```python
from build123d import *

# Parameters (mm, degrees)
SKETCH1_R           = 1.9
SKETCH1_R_2         = 1.2
BOSS_EXTRUDE1_DEPTH = 3.5
SKETCH2_R           = 5.9
SKETCH2_R_2         = 4.9
BOSS_EXTRUDE2_DEPTH = 1.5
BOSS_EXTRUDE3_DEPTH = 0.125
CIRPATTERN1_COUNT   = 3


with BuildPart() as part:
    # Sketch1 → Boss-Extrude1 (new body)
    with BuildSketch(Plane.XY):
        Circle(SKETCH1_R)
        Circle(SKETCH1_R_2, mode=Mode.SUBTRACT)
    extrude(amount=BOSS_EXTRUDE1_DEPTH)



with BuildPart() as body_2:
    # Sketch2 → Boss-Extrude2 (new body)
    with BuildSketch(Plane.XY.offset(3.5)):
        Circle(SKETCH2_R)
        Circle(SKETCH2_R_2, mode=Mode.SUBTRACT)
    extrude(amount=-BOSS_EXTRUDE2_DEPTH)


with BuildPart() as part_1:
    add(part.part)

    add(body_2.part)  # Boss-Extrude3 merges body 2
    # Sketch7 → Boss-Extrude3 (add, symmetric)
    with BuildSketch(Plane(origin=(0, 0, 0), x_dir=(0, 0, -1), z_dir=(1, 0, 0))):
        Polygon((-3.498505426, 1.898798754), (-3.498505426, 4.906659039), (-2.003497041, 4.906659039), (0, 1.898798754), (0, 1.698798754), (-3.498505426, 1.698798754), align=None)
    boss_extrude3 = extrude(amount=BOSS_EXTRUDE3_DEPTH, both=True)

    # CirPattern1: Boss-Extrude3 ×3 about axis
    cirpattern1_axis = Axis((0, 0, 0), (0, 0, 1))
    for i in range(1, CIRPATTERN1_COUNT):
        add(boss_extrude3.rotate(cirpattern1_axis, i * 360 / CIRPATTERN1_COUNT))


solid = part_1.part
```
Work out the finished part from the listing and answer in its coordinate system (mm). A direction names the side the tool comes from. Coordinates: 2 decimals unless noted, no trailing zeros. Order: outer loops, then holes, each group sorted by start corner. A loop starts at its lowest first (then second) coordinate and runs counter-clockwise, first axis right, second up. Notation, with made-up numbers: M 89,77.25 L 119,77.25 A13 ccw 119,89.25 Z; hole C 79.25,61.25 d1. An arc over 180 degrees is marked long. Use CSV: the item, a comma, the result in double quotes.
1) Section C-C on z = 0.65 is taken. Write down the section's boundary in (x, y) (3 decimals).
Worked out:
outline,"M -2.552,-1.329 L -2.427,-1.546 L -1.579,-1.056 A1.9 ccw 1.579,-1.056 L 2.427,-1.546 L 2.552,-1.329 L 1.704,-0.84 A1.9 ccw 0.125,1.896 L 0.125,2.875 L -0.125,2.875 L -0.125,1.896 A1.9 ccw -1.704,-0.84 Z; hole C 0,0 d2.4"
2) Section A-A on y = 2.25 is taken. Count the separate pieces of the cut face and the enclosed holes in it, plus the area to 3 significant figures.
Worked out:
separate pieces,"3"
enclosed holes,"0"
area,"4.12 mm^2"
3) Consider line 1 (Y direction, x = 0, z = 2.7); line 2 (Y direction, x = -1, z = 2.95); line 3 (X direction, y = -1.5, z = 1.5). Determine where each line is inside the solid, lowest interval first. Write a range as [from, to].
Worked out:
line 1,"y = [-5.9, -4.9], [-1.9, -1.2], [1.2, 5.9]"
line 2,"y = [-5.81, -4.8], [-1.62, -0.66], [0.66, 1.62], [4.8, 5.81]"
line 3,"x = [-2.85, -2.35], [-1.17, 1.17], [2.35, 2.85]"
4) Determine the mould class of faces 1 (the face through (-5.894, 0.259, 2.76)), 2 (the face through (-1.9, 0.08, 1.73)), 3 (the face through (1, 5, 2)) for opening direction X: released by +X, released by -X, zero draft, split by the parting line, or undercut.
Worked out:
face 1,"split by the parting line"
face 2,"undercut"
face 3,"zero draft"
5) Section B-B on x = -4.5 is taken. Write down the section's boundary in (y, z).
Worked out:
outline,"M -3.82,2 L -1.94,2 L -1.94,3.5 L -3.82,3.5 Z; M 1.94,2 L 3.82,2 L 3.82,3.5 L 1.94,3.5 Z"
6) Section D-D on y = -4.25 is taken. Write down the section's boundary in (x, z), plus the area to 3 significant figures.
Worked out:
outline,"M -4.09,2 L -2.44,2 L -2.44,3.5 L -4.09,3.5 Z; M 2.44,2 L 4.09,2 L 4.09,3.5 L 2.44,3.5 Z"
area,"4.96 mm^2"
7) Flat-ended cylindrical pins translate along their axes: pin 1 Ø2 at (x, z) = (-2.5, 2) entering from +Y; pin 2 Ø1.5 at (y, z) = (3.5, 1) entering from +X (3 decimals). Find the tip coordinate at first contact, or state that the pin passes through.
Worked out:
pin 1,"stops at y = 5.71"
pin 2,"stops at x = 0.125"
8) For faces 4 (the face through (1, 1, 0)), 5 (the face through (-0.125, 3, 2)), determine the directions among +Z, -Z, +X, -X, +Y, -Y from which every point of the face is accessible in a straight line to the end or side of a thin tool.
Worked out:
face 4,"-Z, +X, -X, +Y, -Y"
face 5,"+Z, -Z"
